Here's the drawing with two shaded views (mm, measured from the low corner). I have some questions. A direction names the side the tool comes from. Give positions to 0.01 mm unless a question says otherwise; leave off trailing zeros. Loops run counter-clockwise (first coordinate to the right, second up) from the corner with the lowest first, then second, coordinate; pieces in that order, holes last. Notation, with made-up numbers: (38.25, 47.5) - (67.25, 47.5) arc R26 ccw to (67.25, 79.5) - close; hole circle Ø5 at (35, 33.5). An arc over 180 degrees is marked (long way). Use one line per item in the form item = value.
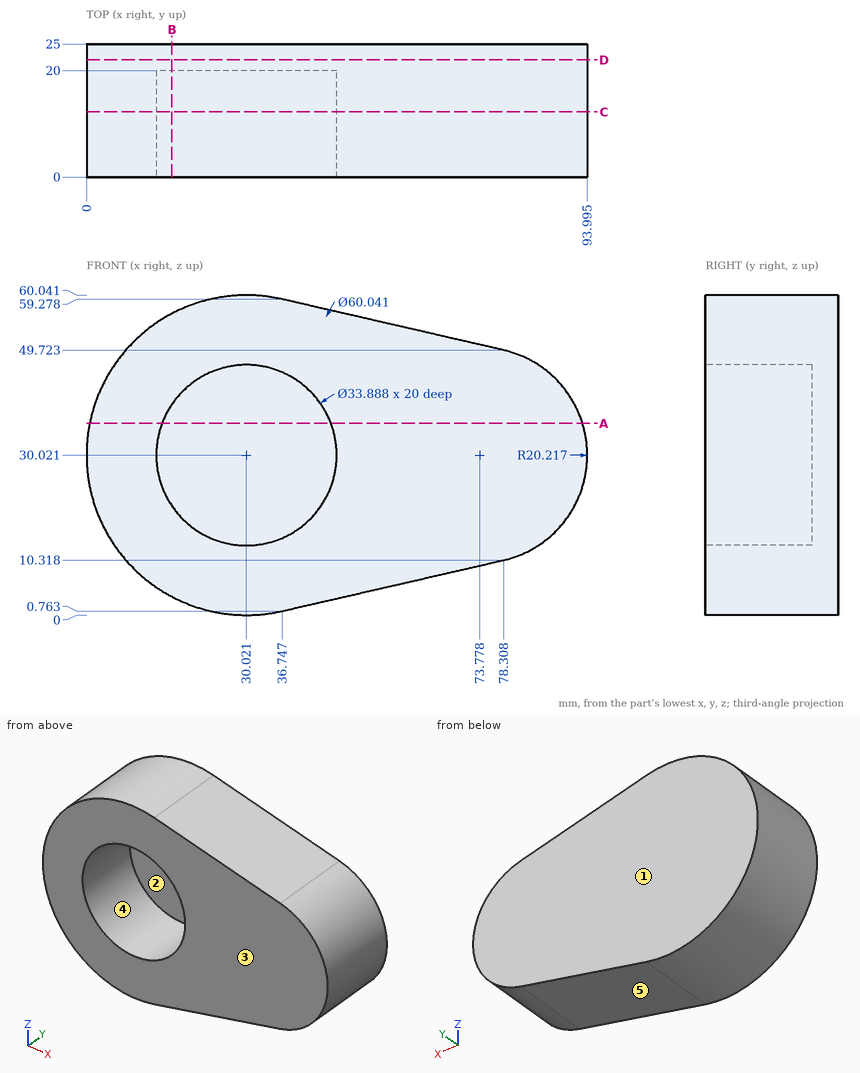
(1) If we section it at C-C (y = 12.25): List the corners of the cut face in (x, z) for me (1 decimal), plus the area to 3 significant figures.
Geometry says:
outline = (36.7, 0.8) - (78.3, 10.3) arc R20.2 ccw to (78.3, 49.7) - (36.7, 59.3) arc R30 ccw (long way) to start; hole circle Ø33.9 at (30, 30)
area = 3,410 mm²
(2) For P1, Ø12, axis at x = 69.5, y = 13.5, coming from the +Z side; P2, Ø8, axis at y = 22.5, z = 38.5, coming from the -X side; P3, Ø1, axis at x = 84, z = 11.5, coming from the +Y side; P4, Ø17, axis at x = 24.5, z = 25, coming from the -Y side, each with a flat end and sliding along its axis, tell me the tip position at first contact or that it passes through.
Geometry says:
P1 = 53.13
P2 = 0.34
P3 = through
P4 = 20
(3) If we section it at A-A (z = 36): List the corners of the cut face in (x, y) for me (1 decimal).
Geometry says:
outline = (0.6, 0) - (14.2, 0) - (14.2, 20) - (45.9, 20) - (45.9, 0) - (93.1, 0) - (93.1, 25) - (0.6, 25) - close
(4) For the marked faces 1 and 2, which set-ups out of +Z, -Z, +X, -X, +Y, -Y let a thin tool reach every point of the face, with its end or its side?
Geometry says:
face_1 = +Z, -Z, +X, -X, +Y
face_2 = -Y
(5) If I drill on probe 1 along X at (y, z) = (7, 30) (1 decimal); probe 2 along Y at (x, z) = (45, 31); probe 3 along X at (y, z) = (11, 14.5) (1 decimal), over which ranges is the centre line in solid material (lowest first)?
Geometry says:
probe_1 = 0 to 13.1, 47 to 94
probe_2 = 20 to 25
probe_3 = 4.3 to 23.2, 36.8 to 86.7
(6) Thinking about a two-plate mould opening in X: for the marked faces 3, 4 and 5, which applies, pulls with the +X half, pulls with the -X half, needs draft (parallel to the pull), parting line crosses it, or undercut?
Geometry says:
face_3 = needs draft
face_4 = undercut
face_5 = pulls with the +X half
(7) If we section it at D-D (y = 22): List the corners of the cut face in (x, z) for me, plus the area to 3 significant figures.
Geometry says:
outline = (36.75, 0.76) - (78.31, 10.32) arc R20.22 ccw to (78.31, 49.72) - (36.75, 59.28) arc R30.02 ccw (long way) to start
area = 4,310 mm²
(8) If we section it at B-B (x = 16): List the corners of the cut face in (y, z) for me (1 decimal), plus the area to 3 significant figures.
Geometry says:
outline = (0, 3.5) - (25, 3.5) - (25, 56.6) - (0, 56.6) - (0, 39.5) - (20, 39.5) - (20, 20.5) - (0, 20.5) - close
area = 947 mm²
